Geometry: final body of the model. Coordinates: model frame, mm. Face numbers are marked on the shaded views. A direction names the side the tool comes from. Give positions to 0.01 mm unless a question says otherwise; leave off trailing zeros. Write each loop counter-clockwise with the first axis right and the second up, starting at its lowest first coordinate (ties: lowest second). Pieces come first, ordered by that corner, then holes.
Q1. Line query: L1, parallel to X at y = 0.35, z = 2.25; L2, parallel to X at y = 3.8, z = 0.25; L3, parallel to Z at x = 22.5, y = 2.45. Output: solid intervals per line, ascending.
Q2. Cut plane D-D on x = 22. Return the cut outline in (y, z).
Q3. Cut plane A-A on z = 0.5. Return the cut outline in (x, y), plus the area to 3 significant figures.
Q4. Draft query along X for the marked faces 3, 4 and 5. Return one class per face: pulls with the +X half, pulls with the -X half, needs draft (parallel to the pull), parting line crosses it, or undercut.
Q5. Pin query (flat end, axial travel): pin 1 (2 mm diameter, centred on x = 23, y = 1, fed in from +Z); pin 2 (2 mm diameter, centred on y = 3, z = 1, fed in from -X). Return the tip coordinate at first contact, or that it passes through.
Q6. Reachability of the marked faces 1 and 2 from +Z, -Z, +X, -X, +Y, -Y: full face, straight path, thin tool, end or side. Return the list, or none.
Q7. Cut plane C-C on z = -1.25. Return the cut outline in (x, y), plus the area to 3 significant figures.
Autodesk Inventor part; units mm, degrees
ref_plane "YZ Plane" through (0, 0, 0) normal (1, 0, 0) x (0, 1, 0)
ref_plane "XZ Plane" through (0, 0, 0) normal (0, 1, 0) x (-1, 0, 0)
ref_plane "XY Plane" through (0, 0, 0) normal (0, 0, 1) x (1, 0, 0)
sketch "Skizze5" plane through (0, 0, 0) normal (0, 1, 0) x (-1, 0, 0)
  line L0 (-17.5, 0) -> (-25, 0)
  line L1 (-31, -2) -> (-31, -3)
  line L2 (-31, -3) -> (0, -3)
  line L3 (0, -3) -> (0, 3)
  line L4 (-31, -2) -> (-26, 3)
  line L5 (-26, 3) -> (-25, 3)
  line L6 (-25, 3) -> (-25, 0)
  line L7 (-17.5, 0) -> (-17.5, 3)
  line L8 (-17.5, 3) -> (0, 3)
  point P0 (0, 0)
  point P1 (0, 0)
  dimension "d33" = 3
  dimension "d34" = 45
  dimension "d35" = 1
  dimension "d36" = 1
  dimension "d37" = 3
  dimension "d38" = 6
  dimension "d39" = 7.5
  dimension "d40" = 17.5
extrude "Extrusion4" add sketch "Skizze5" along normal blind 4.1
fillet "Rundung5" radius 1 1 edges at (25, 2.05, 3)
properties part number "P_Wing_Mountingplate_pin"
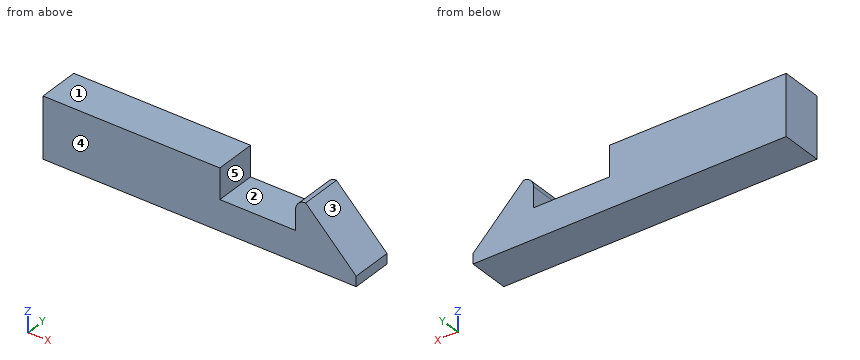
Data:
1. L1: x = 0 to 17.5, 25.03 to 26.75
1. L2: x = 0 to 17.5, 25 to 28.75
1. L3: z = -3 to 0
2. outline: (0, -3) - (4.1, -3) - (4.1, 0) - (0, 0) - close
3. outline: (0, 0) - (17.5, 0) - (17.5, 4.1) - (0, 4.1) - close; (25, 0) - (28.5, 0) - (28.5, 4.1) - (25, 4.1) - close
3. area: 86.1 mm2
4. face 3: pulls with the +X half
4. face 4: needs draft
4. face 5: undercut
5. pin 1: stops at z = 0
5. pin 2: stops at x = 0
6. face 1: +Z, +X, -X, +Y, -Y
6. face 2: +Z, +Y, -Y
7. outline: (0, 0) - (30.25, 0) - (30.25, 4.1) - (0, 4.1) - close
7. area: 124 mm2
